For this review, take the finished solid that the model builds, in its own axes (mm). Face numbers are marked on the shaded views. A direction names the side the tool comes from. Give positions to 0.01 mm unless a question says otherwise; leave off trailing zeros.
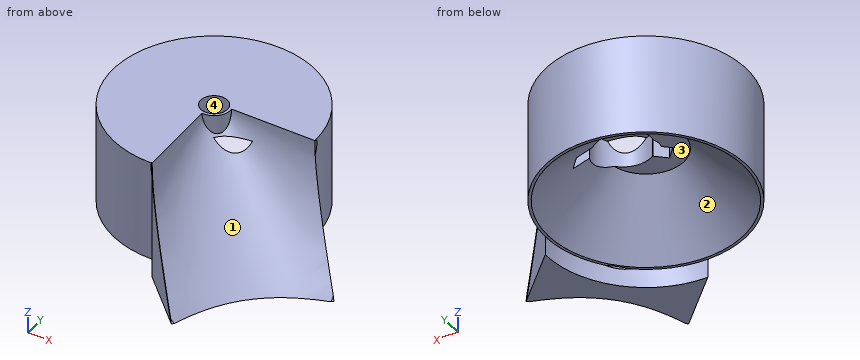
```python
from build123d import *

# Parameters (mm, degrees)
BOX039_W                    = 44
BOX039_H                    = 8
BOX039_DEPTH                = 80
BOX039_PLACEMENT_ANGLE      = 42
CYLINDER023_R               = 1
CYLINDER023_DEPTH           = 10
CYLINDER023_PLACEMENT_ANGLE = 45
CYLINDER024_R               = 1
CYLINDER024_DEPTH           = 10
CYLINDER024_PLACEMENT_ANGLE = 45
CYLINDER022_R               = 15
CYLINDER022_DEPTH           = 80
CYLINDER022_PLACEMENT_ANGLE = 39
CYLINDER026_R               = 8.5
CYLINDER026_DEPTH           = 45
BOX038_W                    = 100
BOX038_H                    = 200
BOX038_DEPTH                = 50
BOX038_PITCH_ANGLE          = 60
BOX038_PLACEMENT_ANGLE      = -45
BOX041_W                    = 100
BOX041_H                    = 100
BOX041_DEPTH                = 100
BOX041_PLACEMENT_ANGLE      = 45
BOX042_W                    = 100
BOX042_H                    = 100
BOX042_DEPTH                = 100
BOX042_PLACEMENT_ANGLE      = 45
BOX043_W                    = 200
BOX043_H                    = 200
BOX043_DEPTH                = 200
CONE008_ANGLE               = 180
CONE008_ROLL_ANGLE          = -90
CONE008_PLACEMENT_ANGLE     = -135
CONE007_ANGLE               = 180
CONE007_ROLL_ANGLE          = -90
CONE007_PLACEMENT_ANGLE     = -135
CYLINDER027_R               = 53
CYLINDER027_DEPTH           = 60
BOX044_W                    = 38
BOX044_H                    = 75
BOX044_DEPTH                = 63
BOX044_PLACEMENT_ANGLE      = 45
CYLINDER025_R               = 53
CYLINDER025_DEPTH           = 53
TUBE018_R                   = 8.5
TUBE018_R_2                 = 7
TUBE018_DEPTH               = 53


with BuildPart() as cube039:
    # Box039 → Box039 (new body)
    with BuildSketch(Plane.XY):
        with Locations((22, 4)):
            Rectangle(BOX039_W, BOX039_H)
    extrude(amount=BOX039_DEPTH)


with BuildPart() as cube039_1:
    # Box039 placement: moved
    add(cube039.part.moved(Location((-5.13, -11.9828, -91))).rotate(Axis((-5.13, -11.9828, -91), (0, 0, 1)), BOX039_PLACEMENT_ANGLE))


with BuildPart() as cone009:
    # Cone009 → Cone009 (revolve)
    with BuildSketch(Plane(origin=(0, 0, -53), x_dir=(1, 0, 0), z_dir=(0, -1, 0))):
        Polygon((0, 0), (51.5, 0), (20, 29), (0, 29), align=None)
    revolve(axis=Axis((0, 0, -53), (0, 0, 1)))


with BuildPart() as cylinder023:
    # Cylinder023 → Cylinder023 (new body)
    with BuildSketch(Plane.XY):
        Circle(CYLINDER023_R)
    extrude(amount=CYLINDER023_DEPTH)


with BuildPart() as cylinder023_1:
    # Cylinder023 placement: moved
    add(cylinder023.part.moved(Location((-18.38, -7.07107, -11))).rotate(Axis((-18.38, -7.07107, -11), (0, 0, 1)), CYLINDER023_PLACEMENT_ANGLE))


with BuildPart() as cylinder024:
    # Cylinder024 → Cylinder024 (new body)
    with BuildSketch(Plane.XY):
        Circle(CYLINDER024_R)
    extrude(amount=CYLINDER024_DEPTH)


with BuildPart() as cylinder024_1:
    # Cylinder024 placement: moved
    add(cylinder024.part.moved(Location((22.49, 18.3848, -11))).rotate(Axis((22.49, 18.3848, -11), (0, 0, 1)), CYLINDER024_PLACEMENT_ANGLE))


with BuildPart() as fusion009012:
    # Cylinder022 → Cylinder022 (new body)
    with BuildSketch(Plane.XY):
        Circle(CYLINDER022_R)
    extrude(amount=CYLINDER022_DEPTH)


with BuildPart() as fusion009012_1:
    # Cylinder022 placement: moved
    add(fusion009012.part.moved(Location((8.58, 5.90251, -91))).rotate(Axis((8.58, 5.90251, -91), (0, 0, 1)), CYLINDER022_PLACEMENT_ANGLE))

    # Fusion009012: union Cube039, Cone009, Cylinder023, Cylinder024
    add(cube039_1.part)
    add(cone009.part)
    add(cylinder023_1.part)
    add(cylinder024_1.part)


with BuildPart() as cylinder026:
    # Cylinder026 → Cylinder026 (new body)
    with BuildSketch(Plane.XY.offset(-43)):
        Circle(CYLINDER026_R)
    extrude(amount=CYLINDER026_DEPTH)


with BuildPart() as cube038:
    # Box038 → Box038 (new body)
    with BuildSketch(Plane.XY):
        with Locations((50, 100)):
            Rectangle(BOX038_W, BOX038_H)
    extrude(amount=BOX038_DEPTH)


with BuildPart() as cube038_1:
    # Box038 pitch: moved
    add(cube038.part.rotate(Axis((0, 0, 0), (0, 1, 0)), BOX038_PITCH_ANGLE))


with BuildPart() as cube038_2:
    # Box038 placement: moved
    add(cube038_1.part.moved(Location((-38.183766, -91.923882, 0))).rotate(Axis((-38.183766, -91.923882, 0), (0, 0, 1)), BOX038_PLACEMENT_ANGLE))


with BuildPart() as cube041:
    # Box041 → Box041 (new body)
    with BuildSketch(Plane.XY):
        with Locations((50, 50)):
            Rectangle(BOX041_W, BOX041_H)
    extrude(amount=BOX041_DEPTH)


with BuildPart() as cube041_1:
    # Box041 placement: moved
    add(cube041.part.moved(Location((-71.320657, -123.15444, -92))).rotate(Axis((-71.320657, -123.15444, -92), (0, 0, -1)), BOX041_PLACEMENT_ANGLE))


with BuildPart() as cube042:
    # Box042 → Box042 (new body)
    with BuildSketch(Plane.XY):
        with Locations((50, 50)):
            Rectangle(BOX042_W, BOX042_H)
    extrude(amount=BOX042_DEPTH)


with BuildPart() as cube042_1:
    # Box042 placement: moved
    add(cube042.part.moved(Location((53.030932, 0.040624, -92))).rotate(Axis((53.030932, 0.040624, -92), (0, 0, -1)), BOX042_PLACEMENT_ANGLE))


with BuildPart() as cube043:
    # Box043 → Box043 (new body)
    with BuildSketch(Plane(origin=(-111, -128, -263), x_dir=(1, 0, 0), z_dir=(0, 0, 1))):
        with Locations((100, 100)):
            Rectangle(BOX043_W, BOX043_H)
    extrude(amount=BOX043_DEPTH)


with BuildPart() as fusion009014:
    # Cone008 → Cone008 (revolve)
    with BuildSketch(Plane.XZ):
        Polygon((0, 0), (2, 0), (78, 80), (0, 80), align=None)
    revolve(axis=Axis((0, 0, 0), (0, 0, 1)), revolution_arc=CONE008_ANGLE)


with BuildPart() as fusion009014_1:
    # Cone008 roll: moved
    add(fusion009014.part.rotate(Axis((0, 0, 0), (1, 0, 0)), CONE008_ROLL_ANGLE))


with BuildPart() as fusion009014_2:
    # Cone008 placement: moved
    add(fusion009014_1.part.rotate(Axis((0, 0, 0), (0, 0, 1)), CONE008_PLACEMENT_ANGLE))

    # Fusion009014: union Cube041, Cube042, Cube043
    add(cube041_1.part)
    add(cube042_1.part)
    add(cube043.part)


with BuildPart() as obj1:
    # Cone007 → Cone007 (revolve)
    with BuildSketch(Plane.XZ):
        Polygon((0, 0), (2, 0), (80, 80), (0, 80), align=None)
    revolve(axis=Axis((0, 0, 0), (0, 0, 1)), revolution_arc=CONE007_ANGLE)


with BuildPart() as obj1_1:
    # Cone007 roll: moved
    add(obj1.part.rotate(Axis((0, 0, 0), (1, 0, 0)), CONE007_ROLL_ANGLE))


with BuildPart() as obj1_2:
    # Cone007 placement: moved
    add(obj1_1.part.rotate(Axis((0, 0, 0), (0, 0, 1)), CONE007_PLACEMENT_ANGLE))


with BuildPart() as cut009009:
    # Cut009017 base: copy of obj1
    add(obj1_2.part)

    # Cut009017: cut Fusion009014
    add(fusion009014_2.part, mode=Mode.SUBTRACT)

    # Cut009009: cut Cube038
    add(cube038_2.part, mode=Mode.SUBTRACT)


with BuildPart() as cylinder027:
    # Cylinder027 → Cylinder027 (new body)
    with BuildSketch(Plane.XY.offset(-63)):
        Circle(CYLINDER027_R)
    extrude(amount=CYLINDER027_DEPTH)


with BuildPart() as cut009012:
    # Box044 → Box044 (new body)
    with BuildSketch(Plane.XY):
        with Locations((19, 37.5)):
            Rectangle(BOX044_W, BOX044_H)
    extrude(amount=BOX044_DEPTH)


with BuildPart() as cut009012_1:
    # Box044 placement: moved
    add(cut009012.part.moved(Location((-0.609979, -52.443762, -63))).rotate(Axis((-0.609979, -52.443762, -63), (0, 0, -1)), BOX044_PLACEMENT_ANGLE))

    # Cut009012: cut Cylinder027
    add(cylinder027.part, mode=Mode.SUBTRACT)


with BuildPart() as cut009010:
    # Cylinder025 → Cylinder025 (new body)
    with BuildSketch(Plane.XY.offset(-53)):
        Circle(CYLINDER025_R)
    extrude(amount=CYLINDER025_DEPTH)

    # Fusion009013: union Cut009012
    add(cut009012_1.part)

    # Cut009011: cut obj1
    add(obj1_2.part, mode=Mode.SUBTRACT)

    # Fusion009011: union Cut009009
    add(cut009009.part)

    # Cut009010: cut Cylinder026
    add(cylinder026.part, mode=Mode.SUBTRACT)


with BuildPart() as cut009_middle002:
    # Tube018 → Tube018 (new body)
    with BuildSketch(Plane.XY.offset(-53)):
        Circle(TUBE018_R)
        Circle(TUBE018_R_2, mode=Mode.SUBTRACT)
    extrude(amount=TUBE018_DEPTH)

    # Fusion009010: union Cut009010
    add(cut009010.part)

    # Cut009013: cut Fusion009012
    add(fusion009012_1.part, mode=Mode.SUBTRACT)


solid = cut009_middle002.part
```
Q1. For probe 1 along Z at (x, y) = (29.5, 13); probe 2 along X at (y, z) = (-6, -45); probe 3 along X at (y, z) = (-11.5, -12.5), list the stretches that pass through material, from the lowest coordinate up.
Answers:
probe 1: z = -35.27 to 0
probe 2: x = -52.66 to -42.39, 42.39 to 59.01
probe 3: x = -51.74 to -5.56, -4.59 to 5.26
Q2. For pin 1 Ø3 at (y, z) = (13, -30.5) entering from -X; pin 2 Ø12 at (x, z) = (28.5, -18.5) entering from +Y; pin 3 Ø1.6 at (x, y) = (23, 18.5) entering from -Z, all flat-tipped, find the tip position at first contact; note any pin that passes through.
Answers:
pin 1: stops at x = -51.74
pin 2: stops at y = 47.99
pin 3: stops at z = -11
Q3. Mouldability with a two-part tool opening along Z and no side actions: class the marked faces 1 and 2 as +Z half, -Z half, draft (parallel to the pull), parting line (faces both ways), or undercut.
Answers:
face 1: +Z half
face 2: -Z half
Q4. Machinability: for the marked faces 3 and 4, which of the approach directions +Z, -Z, +X, -X, +Y, -Y give a long, thin tool a straight path to every point of the face, cutting with its end or side? Answer none if there is none.
Answers:
face 3: -Z
face 4: +Z, -Z
